```python
from build123d import *

# Parameters (mm, degrees)
F0_W      = 88
F0_H      = 88
F1_DEPTH  = 25
F3_DEPTH  = 50
F4_T      = -1
F5_W      = 68
F5_H      = 78
F4_FACE_W = 86
F4_FACE_H = 84.2157470514
F6_DEPTH  = 1


with BuildPart() as f1:
    # F0 (on Front) → F1 (new body, symmetric)
    with BuildSketch(Plane.XZ):
        Rectangle(F0_W, F0_H)
    extrude(amount=F1_DEPTH, both=True)

    # F2 (on Right) → F3 (cut, symmetric)
    with BuildSketch(Plane.YZ):
        Polygon((-25, -44), (25, 44), (-25, 44), align=None)
    extrude(amount=F3_DEPTH, both=True, mode=Mode.SUBTRACT)

    # F4
    f4_openings = [f1.faces().sort_by_distance(p)[0] for p in [
        (0, 0, -44),
    ]]
    offset(amount=F4_T, openings=f4_openings)

    # F5 (on face) + F4_face (on face) → F6 (cut)
    with BuildSketch(Plane(origin=(0, 25, 0), x_dir=(-1, 0, 0), z_dir=(0, 1, 0))):
        with Locations((0, -5)):
            Rectangle(F5_W, F5_H)
    with BuildSketch(Plane(origin=(0, 24, -1.8921264743), x_dir=(1, 0, 0), z_dir=(0, -1, 0))):
        Rectangle(F4_FACE_W, F4_FACE_H)
    extrude(amount=-F6_DEPTH, dir=(0, 1, 0), mode=Mode.SUBTRACT)


solid = f1.part
```
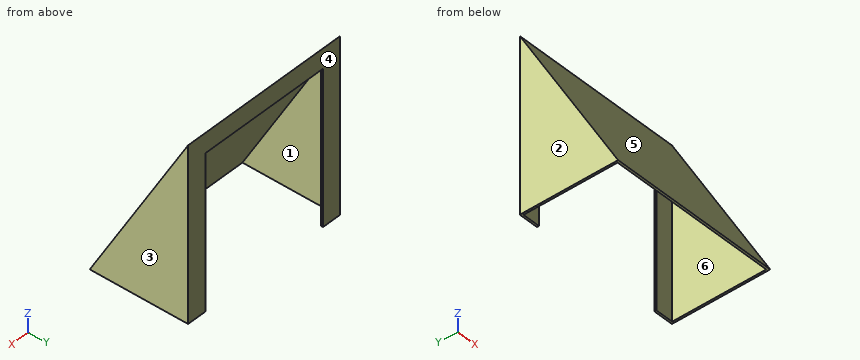
Could you check a few things on this model? Use its own coordinates, in mm. Face numbers are marked on the shaded views. A direction names the side the tool comes from. Round coordinates to 2 decimals unless told otherwise and drop trailing zeros. Loops run counter-clockwise (first coordinate to the right, second up) from the corner with the lowest first, then second, coordinate; pieces in that order, holes last. Notation, with made-up numbers: (-13, 25) - (45, 25) arc R15 ccw to (45, 51) - close; hole circle Ø4 at (29, -23.75). An arc over 180 degrees is marked (long way). Answer as CSV lines item,"result".
1. Please list where these lines run through material, in increasing order: line 1 along X through (y, z) = (4, -39); line 2 along Y through (x, z) = (-36, 3); line 3 along Z through (x, y) = (36.5, 1.5). Write a range as [from, to].
Filled in:
line 1,"x = [-44, -43], [43, 44]"
line 2,"y = [1.7, 2.85], [24, 25]"
line 3,"z = [0.62, 2.64]"
2. For pin 1 Ø4 at (x, z) = (22, -11.5) entering from +Y; pin 2 Ø12 at (x, y) = (2.5, 16.5) entering from +Z; pin 3 Ø0.5 at (x, y) = (-12.5, 23.5) entering from -Z, each with a flat end and sliding along its axis, tell me the tip position at first contact or that it passes through.
Filled in:
pin 1,"stops at y = -4.25"
pin 2,"stops at z = 39.6"
pin 3,"stops at z = 40.22"
3. I want a section at D-D on z = 32.5. List the corners of the cut face in (x, y) for me.
Filled in:
outline,"(-44, 18.47) - (44, 18.47) - (44, 25) - (34, 25) - (34, 24) - (43, 24) - (43, 19.62) - (-43, 19.62) - (-43, 24) - (-34, 24) - (-34, 25) - (-44, 25) - close"
4. I want a section at A-A on x = 0.5. List the corners of the cut face in (y, z) for me, then the cut area to 3 significant figures.
Filled in:
outline,"(-25, -44) - (-23.85, -44) - (23, 38.46) - (23, 40.22) - (24, 40.22) - (24, 34) - (25, 34) - (25, 44) - close"
area,"106 mm^2"
5. I want a section at B-B on z = -28. List the corners of the cut face in (x, y) for me.
Filled in:
outline,"(-44, -15.91) - (44, -15.91) - (44, 25) - (34, 25) - (34, 24) - (43, 24) - (43, -14.76) - (-43, -14.76) - (-43, 24) - (-34, 24) - (-34, 25) - (-44, 25) - close"
6. I want a section at C-C on y = 2.5. List the corners of the cut face in (x, z) for me.
Filled in:
outline,"(-44, -44) - (-43, -44) - (-43, 2.38) - (43, 2.38) - (43, -44) - (44, -44) - (44, 4.4) - (-44, 4.4) - close"
7. On a 3-axis mill with a long thin cutter (end or side, diameter ignored), from which of +Z, -Z, +X, -X, +Y, -Y can I reach the whole of each face in a straight line? I mean the marked faces 1 and 2. Say none if no direction works.
Filled in:
face 1,"-Z"
face 2,"+Z, -Z, -X, +Y, -Y"
8. We'd pull the mould along Y, two halves only. Please class the marked faces 3, 4, 5 and 6: +Y half, -Y half, draft (parallel to the pull), parting line (faces both ways), or undercut.
Filled in:
face 3,"draft"
face 4,"+Y half"
face 5,"-Y half"
face 6,"undercut"
